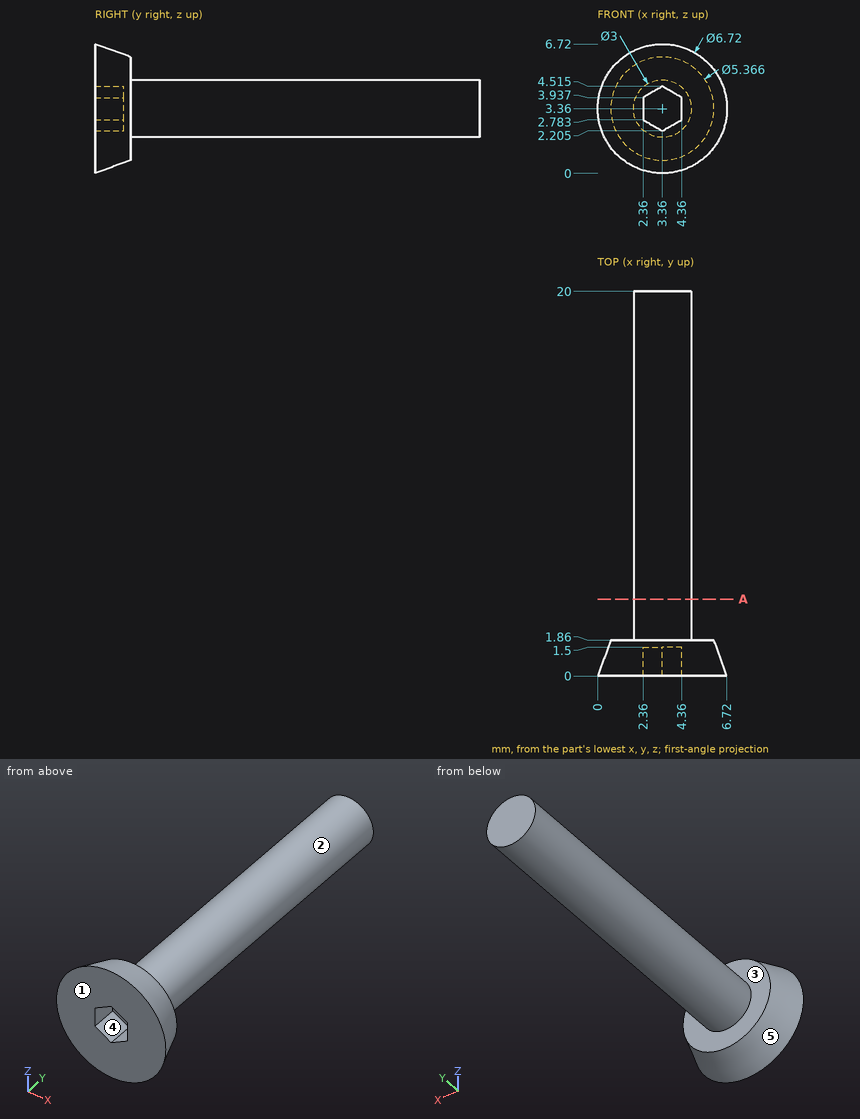
Here's the drawing with two shaded views (mm, measured from the low corner). I have some questions. A direction names the side the tool comes from. Coordinates: 2 decimals unless noted, no trailing zeros. Order: outer loops, then holes, each group sorted by start corner. A loop starts at its lowest first (then second) coordinate and runs counter-clockwise, first axis right, second up. Notation, with made-up numbers: (4.5, -11.5) -> (57.5, -11.5) arc R13 cw to (57.5, -0.5) -> close; hole circle Ø7 at (87.5, -36.75). An arc over 180 degrees is marked (long way). Write each question's results on one line, items separated by ' | '.
Item 1: Which directions (+Z, -Z, +X, -X, +Y, -Y) give clear straight access to the entire face, cutting with the end or side of a thin tool? Please do the marked faces 1 and 2.
Results are:
face 1: +Z, -Z, +X, -X, -Y | face 2: +Y
Item 2: If I drill on line 1 along Y through (x, z) = (1.5, 2.25); line 2 along Y through (x, z) = (3.75, 4.25); line 3 along Z through (x, y) = (3, 17.75), over which ranges is the centre line in solid material (lowest first)?
Results are:
line 1: 0 to 1.86 | line 2: 1.5 to 20 | line 3: 1.9 to 4.82
Item 3: I'm going to push flat-ended pins straight in: pin 1 Ø0.9 at (y, z) = (1, 3.5) entering from +X; pin 2 Ø4 at (y, z) = (6.5, 6) entering from -X; pin 3 Ø1 at (x, y) = (4.5, 10) entering from +Z. Where does each tip first touch, or does it pass through?
Results are:
pin 1: x = 6.52 | pin 2: x = 2 | pin 3: z = 4.72
Item 4: I want a section at A-A, the plane y = 4. Write out the boundary of the cut face in (x, z).
Results are:
outline: circle Ø3 at (3.36, 3.36)
Item 5: If we mould it in two halves opening along Z, with no side actions, what happens to the marked faces 3, 4 and 5? For each: +Z half, -Z half, draft (parallel to the pull), parting line (faces both ways), or undercut.
Results are:
face 3: draft | face 4: undercut | face 5: parting line
